Design review of the part built by this model. Coordinates are the model's own, in mm. Coordinates: 2 decimals unless noted, no trailing zeros. Loops run counter-clockwise (first coordinate to the right, second up) from the corner with the lowest first, then second, coordinate; pieces in that order, holes last.
Q1. Add section B-B on z = 1.75. Give the boundary of the cut face in (x, y) (1 decimal).
Q2. Add section D-D on x = -21.5. Give the boundary of the cut face in (y, z).
Q3. Wall thickness on probe 1 along X at (y, z) = (-14, -1.45); probe 2 along Y at (x, z) = (1.5, 0.5); probe 3 along Y at (x, z) = (33.54, 1.25): over which ranges is each line inside the solid? List them lowest first.
Q4. Add section A-A on y = 0. Give the boundary of the cut face in (x, z).
Q5. For P1, Ø3, axis at x = -33.54, y = 0, coming from the +Z side; P2, Ø4, axis at x = 0.34, y = -15.33, coming from the -Z side; P3, Ø2, axis at y = -17, z = 1, coming from the -X side; P4, Ø1, axis at y = -11, z = -1.5, coming from the -X side, all flat-tipped, find the tip position at first contact; note any pin that passes through.
Q6. Add section C-C on y = -16. Give the boundary of the cut face in (x, z).
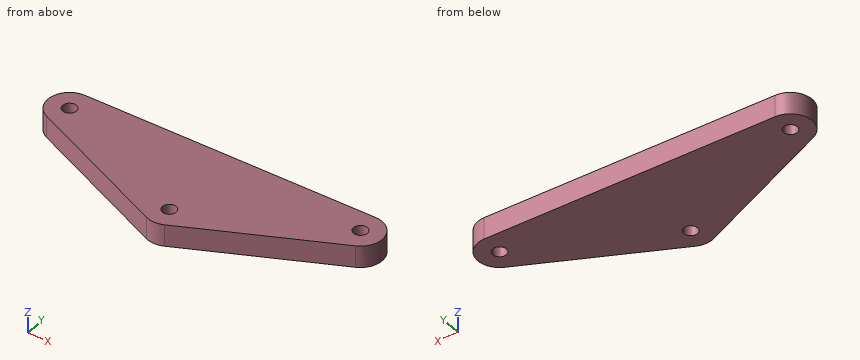
```python
from build123d import *

# Parameters (mm, degrees)
BOSS_EXTRUDE1_DEPTH = 2.5
SKETCH2_R           = 1.5875
CUT_EXTRUDE1_DEPTH  = 44.859171323


with BuildPart() as part:
    # Sketch1 → Boss-Extrude1 (new, symmetric)
    with BuildSketch(Plane.XY):
        with BuildLine():
            Line((-33.54, 5), (33.54, 5))
            ThreePointArc((33.54, 5), (38.423518139, 1.072963462), (35.635934611, -4.539499764))
            Line((35.635934611, -4.539499764), (2.434033336, -19.869165506))
            ThreePointArc((2.434033336, -19.869165506), (0.357155817, -20.329629424), (-1.723171376, -19.885010467))
            Line((-1.723171376, -19.885010467), (-35.601270101, -4.555344726))
            ThreePointArc((-35.601270101, -4.555344726), (-38.42757218, 1.054342537), (-33.54, 5))
        make_face()
    extrude(amount=BOSS_EXTRUDE1_DEPTH, both=True)

    # Sketch2 → Cut-Extrude1 (cut, through all)
    with BuildSketch(Plane.XY.offset(2.5)):
        with Locations((-33.54, 0)):
            Circle(SKETCH2_R)
        with Locations((33.54, 0)):
            Circle(SKETCH2_R)
        with Locations((0.338098725, -15.329665742)):
            Circle(SKETCH2_R)
    extrude(amount=-CUT_EXTRUDE1_DEPTH, mode=Mode.SUBTRACT)


solid = part.part
```
Entries:
1. outline: (-35.6, -4.6) - (-1.7, -19.9) arc R5 ccw to (2.4, -19.9) - (35.6, -4.5) arc R5 ccw to (33.5, 5) - (-33.5, 5) arc R5 ccw to start; hole circle Ø3.2 at (-33.5, 0); hole circle Ø3.2 at (0.3, -15.3); hole circle Ø3.2 at (33.5, 0)
2. outline: (-10.94, -2.5) - (5, -2.5) - (5, 2.5) - (-10.94, 2.5) - close
3. probe 1: x = -14.73 to -0.53, 1.21 to 15.15
3. probe 2: y = -20.19 to -16.41, -14.25 to 5
3. probe 3: y = -5.51 to -1.59, 1.59 to 5
4. outline: (-38.54, -2.5) - (-35.13, -2.5) - (-35.13, 2.5) - (-38.54, 2.5) - close; (-31.95, -2.5) - (31.95, -2.5) - (31.95, 2.5) - (-31.95, 2.5) - close; (35.13, -2.5) - (38.54, -2.5) - (38.54, 2.5) - (35.13, 2.5) - close
5. P1: passes through
5. P2: stops at z = -2.5
5. P3: stops at x = -10.31
5. P4: stops at x = -22.46
6. outline: (-10.31, -2.5) - (-1.1, -2.5) - (-1.1, 2.5) - (-10.31, 2.5) - close; (1.78, -2.5) - (10.81, -2.5) - (10.81, 2.5) - (1.78, 2.5) - close
